Input: part model. Units: mm. Frame: model coordinates. A direction names the side the tool comes from. Round coordinates to 2 decimals unless told otherwise and drop trailing zeros. Loops run counter-clockwise (first coordinate to the right, second up) from the corner with the lowest first, then second, coordinate; pieces in that order, holes last. Notation, with made-up numbers: (-35.75, -1) -> (-9.75, -1) arc R27 cw to (-9.75, 26) -> close; hole circle Ø6 at (36.5, 80.5). An arc over 180 degrees is marked (long way). Answer as a JSON object with one key per item and string values.
Autodesk Inventor part; units mm, degrees
ref_plane "YZ Plane" through (0, 0, 0) normal (1, 0, 0) x (0, 1, 0)
ref_plane "XZ Plane" through (0, 0, 0) normal (0, 1, 0) x (-1, 0, 0)
ref_plane "XY Plane" through (0, 0, 0) normal (0, 0, 1) x (1, 0, 0)
sketch "スケッチ1" plane through (0, 0, 0) normal (0, 0, 1) x (1, 0, 0)
  line L0 (6, -6) -> (-6, -6)
  line L1 (-6, -6) -> (-6, 6)
  line L2 (-6, 6) -> (6, 6)
  line L3 (6, 6) -> (6, -6)
  line L4 (6, -6) -> (-6, 6) construction
  line L5 (-6, -6) -> (6, 6) construction
  point P0 (0, 0)
  dimension "d0" = 12
  dimension "d1" = 12
extrude "押し出し1" add sketch "スケッチ1" along normal blind 4.5
sketch "スケッチ2" plane through (0, 0, 4.5) normal (0, 0, 1) x (1, 0, 0)
  circle A0 centre (0, 0) radius 4
  dimension "d4" = 8
extrude "押し出し2" add sketch "スケッチ2" along normal blind 2
sketch "スケッチ3" plane through (0, 0, 6.5) normal (0, 0, 1) x (1, 0, 0)
  circle A0 centre (0, 0) radius 2.5
  dimension "d7" = 5
extrude "押し出し3" add sketch "スケッチ3" along normal blind 3
properties part number "switch"
1) Section C-C, the plane z = 8. Output: boundary loops of the cut face in (x, y).
Output:
{"outline": "circle Ø5 at (0, 0)"}
2) Ray query, probe 1 along Z at (x, y) = (-5, 0.25); probe 2 along Z at (x, y) = (-2, 2); probe 3 along X at (y, z) = (1.25, 8). Return the intervals inside material, ascending.
Output:
{"probe 1": "z = 0 to 4.5", "probe 2": "z = 0 to 6.5", "probe 3": "x = -2.17 to 2.17"}
3) Reachability of faces 1 (the face through (-0.54, 2.44, 7.98)), 2 (the face through (-6, 0, 2)) from +Z, -Z, +X, -X, +Y, -Y: full face, straight path, thin tool, end or side. Return the list, or none.
Output:
{"face 1": "+Z", "face 2": "+Z, -Z, -X, +Y, -Y"}
4) Section A-A, the plane x = 0. Output: boundary loops of the cut face in (y, z).
Output:
{"outline": "(-6, 0) -> (6, 0) -> (6, 4.5) -> (4, 4.5) -> (4, 6.5) -> (2.5, 6.5) -> (2.5, 9.5) -> (-2.5, 9.5) -> (-2.5, 6.5) -> (-4, 6.5) -> (-4, 4.5) -> (-6, 4.5) -> close"}
5) Contact query for a flat-ended pin moving along its axis: P1, Ø1, axis at x = -3, z = 5.5, coming from the +Y side. Output: stop coordinate, or through.
Output:
{"P1": "stops at y = 3.12"}
6) Section B-B, the plane y = -3. Output: boundary loops of the cut face in (x, z).
Output:
{"outline": "(-6, 0) -> (6, 0) -> (6, 4.5) -> (2.65, 4.5) -> (2.65, 6.5) -> (-2.65, 6.5) -> (-2.65, 4.5) -> (-6, 4.5) -> close"}
